Could you check a few things on this model? Use its own coordinates, in mm. A direction names the side the tool comes from. Round coordinates to 2 decimals unless told otherwise and drop trailing zeros. Loops run counter-clockwise (first coordinate to the right, second up) from the corner with the lowest first, then second, coordinate; pieces in that order, holes last. Notation, with made-up numbers: M 24.25,37 L 53.25,37 A29 ccw 53.25,76 Z; hole C 87,50 d10. An arc over 180 degrees is marked long. Return JSON: item names as keys, results as strings. Group by question number.
```python
from build123d import *

# Parameters (mm, degrees)
BOSS_EXTRUDE1_DEPTH = 6.35
CUT_EXTRUDE3_REACH  = 377.568
SKETCH4_R           = 110.109
SKETCH9_R           = 22.225
CUT_EXTRUDE8_DEPTH  = 376.567629742
SKETCH11_W          = 3.175
SKETCH11_H          = 3.175
CUT_EXTRUDE10_DEPTH = 376.567629742
CUT_EXTRUDE12_DEPTH = 376.567629742
CUT_EXTRUDE15_DEPTH = 376.567629742
CUT_EXTRUDE18_DEPTH = 376.567629742


with BuildPart() as part:
    # Sketch1 → Boss-Extrude1 (new body)
    with BuildSketch(Plane.XY):
        Polygon((279.4, 0), (315.7855, 63.021534659), (234.035835214, 203.2), (-234.035835214, 203.2), (-315.7855, 63.021534659), (-279.4, 0), align=None)
    extrude(amount=BOSS_EXTRUDE1_DEPTH)

    # Sketch4 → Cut-Extrude3 (cut, up to next)
    with BuildSketch(Plane.XY.offset(6.35), mode=Mode.PRIVATE) as cut_extrude3_sk1:
        with Locations((110.49, 127)):
            Circle(SKETCH4_R)
    cut_extrude3_tool1 = extrude(cut_extrude3_sk1.sketch, amount=-CUT_EXTRUDE3_REACH, mode=Mode.PRIVATE) & part.part
    # Sketch4 → Cut-Extrude3 (cut, up to next)
    with BuildSketch(Plane.XY.offset(6.35), mode=Mode.PRIVATE) as cut_extrude3_sk2:
        with Locations((-110.49, 127)):
            Circle(SKETCH4_R)
    cut_extrude3_tool2 = extrude(cut_extrude3_sk2.sketch, amount=-CUT_EXTRUDE3_REACH, mode=Mode.PRIVATE) & part.part
    add(cut_extrude3_tool1.solids().sort_by_distance((110.49, 127, 6.35))[0], mode=Mode.SUBTRACT)
    add(cut_extrude3_tool2.solids().sort_by_distance((-110.49, 127, 6.35))[0], mode=Mode.SUBTRACT)

    # Sketch9 → Cut-Extrude8 (cut, through all)
    with BuildSketch(Plane.XY.offset(6.35)):
        with Locations((252.2855, 37.621534659)):
            Circle(SKETCH9_R)
        with Locations(Location((-252.2855, 37.621534659, 0), (0, 0, 180))):
            Circle(SKETCH9_R)
    extrude(amount=-CUT_EXTRUDE8_DEPTH, mode=Mode.SUBTRACT)

    # Sketch11 → Cut-Extrude10 (cut, through all)
    with BuildSketch(Plane.XY.offset(6.35)):
        with Locations((139.8905, 1.5875)):
            Rectangle(SKETCH11_W, SKETCH11_H)
        with Locations((0, 1.5875)):
            Rectangle(SKETCH11_W, SKETCH11_H)
        with Locations((-139.8905, 1.5875)):
            Rectangle(SKETCH11_W, SKETCH11_H)
    extrude(amount=-CUT_EXTRUDE10_DEPTH, mode=Mode.SUBTRACT)

    # Sketch13 → Cut-Extrude12 (cut, through all)
    with BuildSketch(Plane.XY.offset(6.35)):
        Polygon((-37.517518134, 76.2), (35.644230094, 76.2), (220.599, 127), (220.599, 203.2), (-220.599, 203.2), (-220.599, 127), align=None)
    extrude(amount=-CUT_EXTRUDE12_DEPTH, mode=Mode.SUBTRACT)

    # Sketch16 → Cut-Extrude15 (cut, through all)
    with BuildSketch(Plane(origin=(0, 0, 0), x_dir=(-1, 0, 0), z_dir=(0, 0, -1))):
        with BuildLine():
            Line((-247.674355458, 149.561981252), (-284.88900676, 85.748964754))
            ThreePointArc((-284.88900676, 85.748964754), (-284.909826298, 79.387005073), (-279.403651302, 76.2))
            Line((-279.403651302, 76.2), (-242.189, 76.2))
            ThreePointArc((-242.189, 76.2), (-237.698871939, 78.059871939), (-235.839, 82.55))
            Line((-235.839, 82.55), (-235.839, 146.363016498))
            ThreePointArc((-235.839, 146.363016498), (-240.532121483, 152.493045338), (-247.674355458, 149.561981252))
        make_face()
        with BuildLine():
            Line((242.189, 76.2), (279.403651302, 76.2))
            ThreePointArc((279.403651302, 76.2), (284.909826298, 79.387005073), (284.88900676, 85.748964754))
            Line((284.88900676, 85.748964754), (247.674355458, 149.561981252))
            ThreePointArc((247.674355458, 149.561981252), (240.532121483, 152.493045338), (235.839, 146.363016498))
            Line((235.839, 146.363016498), (235.839, 82.55))
            ThreePointArc((235.839, 82.55), (237.698871939, 78.059871939), (242.189, 76.2))
        make_face()
    extrude(amount=-CUT_EXTRUDE15_DEPTH, mode=Mode.SUBTRACT)

    # Sketch19 → Cut-Extrude18 (cut, through all)
    with BuildSketch(Plane(origin=(0, 0, 0), x_dir=(-1, 0, 0), z_dir=(0, 0, -1))):
        Polygon((-306.188605737, 79.477601033), (-309.387570492, 73.992245575), (-303.243972379, 70.40940505), (-300.045007624, 75.894760508), align=None)
        Polygon((-253.014789274, 171.632766807), (-246.871191161, 168.049926283), (-243.672226407, 173.535281741), (-249.81582452, 177.118122266), align=None)
        Polygon((249.81582452, 177.118122266), (253.014789274, 171.632766807), (246.871191161, 168.049926283), (243.672226407, 173.535281741), align=None)
        Polygon((300.045007624, 75.894760508), (306.188605737, 79.477601033), (309.387570492, 73.992245575), (303.243972379, 70.40940505), align=None)
    extrude(amount=-CUT_EXTRUDE18_DEPTH, mode=Mode.SUBTRACT)


solid = part.part
```
1. If we section it at D-D, the plane x = 181: Please give me the cut outline in (y, z), then the cut area to 3 significant figures.
2. If we section it at B-B, the plane y = 48: Please give me the cut outline in (x, z).
3. On a 3-axis mill with a long thin cutter (end or side, diameter ignored), from which of +Z, -Z, +X, -X, +Y, -Y can I reach the whole of each face in a straight line? I mean faces 1 (the face through (-266.54, 117.21, 3.13)), 2 (the face through (134.64, 19.57, 3.22)). Say none if no direction works.
4. We'd pull the mould along X, two halves only. Please class faces 3 (the face through (-273.484, 30.946, 3.219)), 4 (the face through (-1, 64, 6.35)), 5 (the face through (297.34, 31.07, 3.13)): +X half, -X half, draft (parallel to the pull), parting line (faces both ways), or undercut.
5. I need wall thicknesses on probe 1 along X at (y, z) = (124.5, 2); probe 2 along X at (y, z) = (45, 5); probe 3 along X at (y, z) = (118.5, 5.5). Which ranges of each line are inside material? Lowest first, please.
6. If we section it at A-A, the plane y = 184: Please give me the cut outline in (x, z).
7. I'm going to push flat-ended pins straight in: pin 1 Ø2.5 at (y, z) = (1.5, 3) entering from +X; pin 2 Ø1.6 at (y, z) = (2.5, 4) entering from -X; pin 3 Ø1.6 at (x, z) = (-140.5, 3) entering from -Y (3 decimals). Where does each tip first touch, or does it pass through?
8. If we section it at C-C, the plane z = 4: Give the number of separate pieces and of enclosed holes in the cut face, then the cut area to 3 significant figures.
Geometry results:
{
 "1": {"outline": "M 0,0 L 42.43,0 L 42.43,6.35 L 0,6.35 Z", "area": "269 mm^2"},
 "2": {"outline": "M -307.11,0 L -271.94,0 L -271.94,6.35 L -307.11,6.35 Z; M -232.63,0 L -187.19,0 L -187.19,6.35 L -232.63,6.35 Z; M -33.79,0 L 33.79,0 L 33.79,6.35 L -33.79,6.35 Z; M 187.19,0 L 232.63,0 L 232.63,6.35 L 187.19,6.35 Z; M 271.94,0 L 307.11,0 L 307.11,6.35 L 271.94,6.35 Z"},
 "3": {"face 1": "+Z, -Z", "face 2": "+Z, -Z, +Y"},
 "4": {"face 3": "undercut", "face 4": "draft", "face 5": "+X half"},
 "5": {"probe 1": "-279.93 to -262.29, -235.84 to -220.57, 220.57 to 235.84, 262.29 to 279.93", "probe 2": "-305.38 to -273.25, -231.32 to -183.97, -37.01 to 37.01, 183.97 to 231.32, 273.25 to 305.38", "probe 3": "-283.43 to -265.79, -235.84 to -220.27, 220.27 to 235.84, 265.79 to 283.43"},
 "6": {"outline": "M -245.23,0 L -220.6,0 L -220.6,6.35 L -245.23,6.35 Z; M 220.6,0 L 245.23,0 L 245.23,6.35 L 220.6,6.35 Z"},
 "7": {"pin 1": "x = 280.99", "pin 2": "x = -281.31", "pin 3": "y = 3.175"},
 "8": {"separate pieces": "1", "enclosed holes": "4", "area": "34,300 mm^2"}
}
